For this review, take the finished solid that the model builds, in its own axes (mm). Round coordinates to 2 decimals unless told otherwise and drop trailing zeros. Write each loop counter-clockwise with the first axis right and the second up, starting at its lowest first coordinate (ties: lowest second). Pieces come first, ordered by that corner, then holes.
from build123d import *

# Parameters (mm, degrees)
AUFSATZ_LINEAR_AUSTRAGEN1_DEPTH       = 10
SKIZZE17_R                            = 2.75
SCHNITT_LINEAR_AUSTRAGEN1_DEPTH       = 10
F_10_0_10_DURCHMESSER_BOHRUNG1_D      = 10
F_5_5_5_5_DURCHMESSER_BOHRUNG2_D      = 5.5
F_10_0_10_DURCHMESSER_LANGLOCH2_DEPTH = 10
F_5_5_5_5_DURCHMESSER_LANGLOCH2_DEPTH = 10
F_5_5_5_5_DURCHMESSER_BOHRUNG3_D      = 5.5


# Read off the part's stored shape, not the designer's step: Ø10.0 (10) Durchmesser Langloch2, Ø5.5 (5.5) Durchmesser Langloch2
with BuildPart() as part:
    # Skizze1 → Aufsatz-Linear austragen1 (new body)
    with BuildSketch(Plane.XY):
        Polygon((-40, 681), (-130, 50), (-130, 0), (0, 0), (0, 800), (0, 850), (-25, 850), (-25, 800), (-25, 681), align=None)
    aufsatz_linear_austragen1 = extrude(amount=AUFSATZ_LINEAR_AUSTRAGEN1_DEPTH)

    # Spiegeln1: Aufsatz-Linear austragen1 across plane
    add(aufsatz_linear_austragen1.mirror(Plane(origin=(0, 800, 10), x_dir=(0, 0, 1), z_dir=(1, 0, 0))))

    # Skizze17 → Schnitt-Linear austragen1 (cut)
    with BuildSketch(Plane.XY.offset(10)):
        with Locations((0, 816)):
            Circle(SKIZZE17_R)
        with Locations((0, 784)):
            Circle(SKIZZE17_R)
        with Locations((10, 750.444801834)):
            Circle(SKIZZE17_R)
        with Locations((10, 718.444801834)):
            Circle(SKIZZE17_R)
        with BuildLine():
            Line((-3.535533906, 803.535533906), (25, 832.071067812))
            ThreePointArc((25, 832.071067812), (32.071067812, 832.071067812), (32.071067812, 825))
            Line((32.071067812, 825), (3.535533906, 796.464466094))
            ThreePointArc((3.535533906, 796.464466094), (-3.535533906, 796.464466094), (-3.535533906, 803.535533906))
        make_face()
        with BuildLine():
            Line((6.464466094, 737.98033574), (25, 756.515869646))
            ThreePointArc((25, 756.515869646), (32.071067812, 756.515869646), (32.071067812, 749.444801834))
            Line((32.071067812, 749.444801834), (13.535533906, 730.909267928))
            ThreePointArc((13.535533906, 730.909267928), (6.464466094, 730.909267928), (6.464466094, 737.98033574))
        make_face()
    extrude(amount=-SCHNITT_LINEAR_AUSTRAGEN1_DEPTH, mode=Mode.SUBTRACT)

    # Ø10.0 (10) Durchmesser Bohrung1 (through all)
    with Locations(Plane.XY.offset(10)):
        with Locations((0, 80)):
            Hole(F_10_0_10_DURCHMESSER_BOHRUNG1_D / 2)

    # Ø5.5 (5.5) Durchmesser Bohrung2 (through all)
    with Locations(Plane.XY.offset(10)):
        with Locations((-16, 80), (16, 80)):
            Hole(F_5_5_5_5_DURCHMESSER_BOHRUNG2_D / 2)

    # Ø10.0 (10) Durchmesser Langloch2 outline → Ø10.0 (10) Durchmesser Langloch2 (cut)
    with BuildSketch(Plane.XY):
        with BuildLine():
            Line((20, 168.190997141), (80, 168.190997141))
            ThreePointArc((80, 168.190997141), (85, 173.190997141), (80, 178.190997141))
            Line((80, 178.190997141), (20, 178.190997141))
            ThreePointArc((20, 178.190997141), (15, 173.190997141), (20, 168.190997141))
        make_face()
    extrude(amount=F_10_0_10_DURCHMESSER_LANGLOCH2_DEPTH, mode=Mode.SUBTRACT)

    # Ø5.5 (5.5) Durchmesser Langloch2 outline → Ø5.5 (5.5) Durchmesser Langloch2 (cut)
    with BuildSketch(Plane.XY):
        with BuildLine():
            Line((17.75, 147.940997141), (82.25, 147.940997141))
            ThreePointArc((82.25, 147.940997141), (85, 150.690997141), (82.25, 153.440997141))
            Line((82.25, 153.440997141), (17.75, 153.440997141))
            ThreePointArc((17.75, 153.440997141), (15, 150.690997141), (17.75, 147.940997141))
        make_face()
        with BuildLine():
            Line((17.75, 192.940997141), (82.25, 192.940997141))
            ThreePointArc((82.25, 192.940997141), (85, 195.690997141), (82.25, 198.440997141))
            Line((82.25, 198.440997141), (17.75, 198.440997141))
            ThreePointArc((17.75, 198.440997141), (15, 195.690997141), (17.75, 192.940997141))
        make_face()
    extrude(amount=F_5_5_5_5_DURCHMESSER_LANGLOCH2_DEPTH, mode=Mode.SUBTRACT)

    # Ø5.5 (5.5) Durchmesser Bohrung3 (through all)
    with Locations(Plane.XY.offset(10)):
        with Locations((-34.48740284, 670.074959222), (-71.470822821, 410.780092469), (-119.989782887, 70.608272452)):
            f_5_5_5_5_durchmesser_bohrung3 = Hole(F_5_5_5_5_DURCHMESSER_BOHRUNG3_D / 2)

    # Spiegeln2: Ø5.5 (5.5) Durchmesser Bohrung3 across plane
    add(f_5_5_5_5_durchmesser_bohrung3.mirror(Plane(origin=(0, 0, 0), x_dir=(0, 0, 1), z_dir=(1, 0, 0))), mode=Mode.SUBTRACT)


solid = part.part
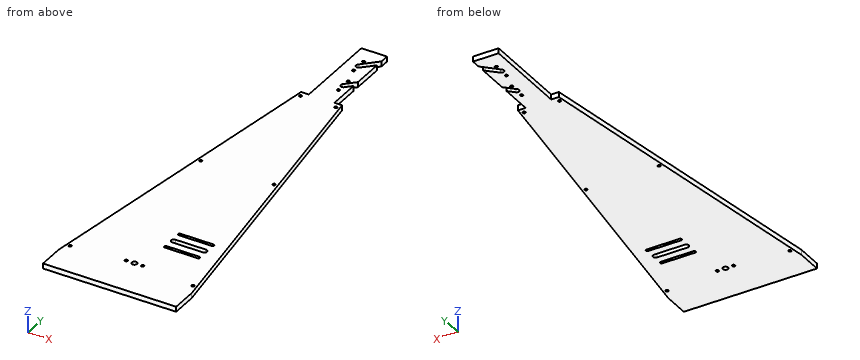
(1) We need section B-B, the plane z = 3.75. State how many separate pieces and enclosed holes the cut face has, and give its area (3 significant figures).
Geometry check:
separate pieces: 1
enclosed holes: 16
area: 126,000 mm2
(2) We need section A-A, the plane x = 96. Give the boundary of the cut face in (y, z).
Geometry check:
outline: (0, 0) - (288.38, 0) - (288.38, 10) - (0, 10) - close
(3) For pin 1 Ø5 at (x, z) = (-33.5, 3.5) entering from +Y; pin 2 Ø3.5 at (x, y) = (119.99, 70.61) entering from -Z; pin 3 Ø5 at (y, z) = (840, 3.5) entering from +X; pin 4 Ø1 at (y, z) = (484, 7.5) entering from -X, all flat-tipped, find the tip position at first contact; note any pin that passes through.
Geometry check:
pin 1: stops at y = 681
pin 2: passes through
pin 3: stops at x = 25
pin 4: stops at x = -68.17
(4) We need section C-C, the plane y = 272. Give the boundary of the cut face in (x, z).
Geometry check:
outline: (-98.34, 0) - (98.34, 0) - (98.34, 10) - (-98.34, 10) - close
(5) For line 1 along Y through (x, z) = (-16, 6.5); line 2 along Y through (x, z) = (0, 6); line 3 along X through (y, z) = (781.5, 5), list the stretches that pass through material, from the lowest coordinate up.
Geometry check:
line 1: y = 0 to 77.25, 82.75 to 850
line 2: y = 0 to 75, 85 to 781.25, 786.75 to 795, 807.07 to 813.25, 818.75 to 850
line 3: x = -25 to -1.15, 1.15 to 25
